```python
from build123d import *

# Parameters (mm, degrees)
BOSS_EXTRUDE1_DEPTH = 12
SKETCH2_R           = 3.375
CUT_EXTRUDE1_DEPTH  = 7


with BuildPart() as part:
    # Sketch1 → Boss-Extrude1 (new body)
    with BuildSketch(Plane.XY):
        Polygon((0, 6.3), (5.4, 6.3), (5.4, 4), (8.5, 4), (8.5, 0), (0, 0), align=None)
    boss_extrude1 = extrude(amount=BOSS_EXTRUDE1_DEPTH)

    # Mirror1: Boss-Extrude1 across plane
    add(boss_extrude1.mirror(Plane(origin=(0, 0, 0), x_dir=(0, 0, 1), z_dir=(1, 0, 0))))

    # Sketch2 → Cut-Extrude1 (cut)
    with BuildSketch(Plane(origin=(0, 6.3, 0), x_dir=(1, 0, 0), z_dir=(0, 1, 0))):
        with Locations((0, -6)):
            Circle(SKETCH2_R)
    extrude(amount=-CUT_EXTRUDE1_DEPTH, mode=Mode.SUBTRACT)


solid = part.part
```
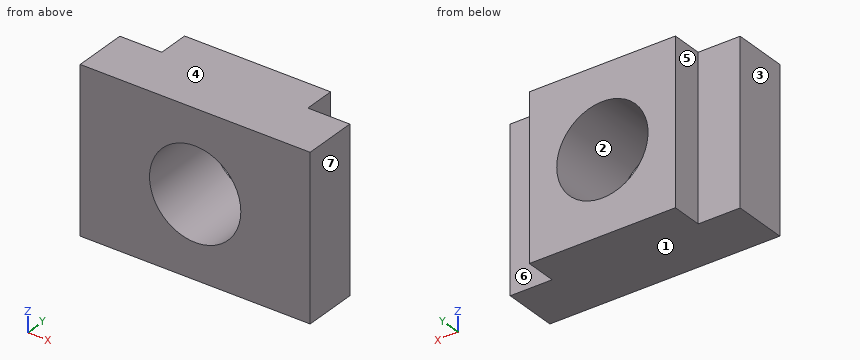
The listing builds one solid part. Answer for the finished solid, in the listing's coordinates (mm). Face numbers are marked on the shaded views. A direction names the side the tool comes from. Round coordinates to 2 decimals unless told otherwise and drop trailing zeros. Loops run counter-clockwise (first coordinate to the right, second up) from the corner with the lowest first, then second, coordinate; pieces in that order, holes last. Notation, with made-up numbers: (38.5, 30) - (58.5, 30) arc R28 cw to (58.5, 52) - close; hole circle Ø9 at (-4.5, -33.75). An arc over 180 degrees is marked (long way). Return JSON: item names as keys, results as strings. Group by question number.
1. Consider probe 1 along Z at (x, y) = (0, 2.75) (3 decimals); probe 2 along X at (y, z) = (4.5, 6) (3 decimals); probe 3 along X at (y, z) = (2.25, 6) (3 decimals). Determine where each line is inside the solid, lowest interval first.
2. Which of the six approach directions +Z, -Z, +X, -X, +Y, -Y give full straight-line access (tool end or side, diameter ignored) to the marked faces 5, 6 and 7?
3. The part is cut by section B-B on z = 6. Determine the outline of the cut face in (x, y) (3 decimals), then the cut area to 3 significant figures.
4. The part is cut by section D-D on z = 1.5. Determine the outline of the cut face in (x, y).
5. The part is cut by section A-A on x = 0. Determine the outline of the cut face in (y, z) (3 decimals).
6. The mould has two halves that part along Z. Classify the marked faces 1, 2, 3 and 4: pulls with the +Z half, pulls with the -Z half, needs draft (parallel to the pull), parting line crosses it, or undercut.
7. Each of these flat-tipped pins is pushed along its axis until it touches: P1, Ø1.5, axis at x = 6.5, z = 5.5, coming from the +Y side; P2, Ø1.8, axis at y = 5, z = 4, coming from the -X side. Where does it stop, or does it pass through?
8. The part is cut by section C-C on y = 5.75. Determine the outline of the cut face in (x, z) (3 decimals), then the cut area to 3 significant figures.
Resolved:
{
 "1": {"probe 1": "z = 0 to 2.625, 9.375 to 12", "probe 2": "x = -5.4 to -3.375, 3.375 to 5.4", "probe 3": "x = -8.5 to -3.375, 3.375 to 8.5"},
 "2": {"face 5": "+Z, -Z, -X, +Y", "face 6": "+Z, -Z, +X, +Y", "face 7": "+Z, -Z, +X, +Y, -Y"},
 "3": {"outline": "(-8.5, 0) - (-3.375, 0) - (-3.375, 6.3) - (-5.4, 6.3) - (-5.4, 4) - (-8.5, 4) - close; (3.375, 0) - (8.5, 0) - (8.5, 4) - (5.4, 4) - (5.4, 6.3) - (3.375, 6.3) - close", "area": "50.3 mm²"},
 "4": {"outline": "(-8.5, 0) - (8.5, 0) - (8.5, 4) - (5.4, 4) - (5.4, 6.3) - (-5.4, 6.3) - (-5.4, 4) - (-8.5, 4) - close"},
 "5": {"outline": "(0, 0) - (6.3, 0) - (6.3, 2.625) - (0, 2.625) - close; (0, 9.375) - (6.3, 9.375) - (6.3, 12) - (0, 12) - close"},
 "6": {"face 1": "pulls with the -Z half", "face 2": "undercut", "face 3": "needs draft", "face 4": "pulls with the +Z half"},
 "7": {"P1": "stops at y = 4", "P2": "stops at x = -5.4"},
 "8": {"outline": "(-5.4, 0) - (5.4, 0) - (5.4, 12) - (-5.4, 12) - close; hole circle Ø6.75 at (0, 6)", "area": "93.8 mm²"}
}
